Read the model definition and answer for the solid it produces. Units are mm, in the model's axes. Face numbers are marked on the shaded views. A direction names the side the tool comes from. Coordinates: 2 decimals unless noted, no trailing zeros. Loops run counter-clockwise (first coordinate to the right, second up) from the corner with the lowest first, then second, coordinate; pieces in that order, holes last. Notation, with made-up numbers: M -39,-20.5 L 12,-20.5 A21 cw 12,1.5 Z; hole C -13,-33.5 d2. An arc over 180 degrees is marked long. Use one line per item in the form item = value. Start each with the question number.
1. The part is cut by section D-D (x = -29). Give the vertices of the cut face in (y, z), plus the area to 3 significant figures.
2. Find the intervals of material crossed by probe 1 along X at (y, z) = (10.25, 8.75); probe 2 along Y at (x, z) = (-38.25, 3.5); probe 3 along X at (y, z) = (11.75, 6.5), in increasing order. Write a range as [from, to].
3. The part is cut by section B-B (x = -38.5). Give the vertices of the cut face in (y, z), plus the area to 3 significant figures.
4. The part is cut by section A-A (y = 12.5). Give the vertices of the cut face in (x, z).
5. A tool of negligible diameter and unlimited length cuts with its end or side. For the marked faces 1 and 2, from which of +Z, -Z, +X, -X, +Y, -Y can it reach the whole face along a straight path? Write none if from no direction.
6. Flat-ended cylindrical pins translate along their axes: pin 1 (2 mm diameter, centred on x = -40.5, y = 9, fed in from -Z); pin 2 (3 mm diameter, centred on y = 1.5, z = 8.5, fed in from +X); pin 3 (4.5 mm diameter, centred on x = -40.41, y = 10.65, fed in from +Z); pin 4 (2 mm diameter, centred on x = -36.5, y = 3.5, fed in from +Z). Find the tip coordinate at first contact, or state that the pin passes through.
7. For a pull along Z with two mould halves and no side action, classify the marked faces 3, 4, 5 and 6 as released by +Z, released by -Z, zero draft, split by the parting line, or undercut.
8. The part is cut by section C-C (z = 2). Give the vertices of the cut face in (x, y).
from build123d import *

# Parameters (mm, degrees)
CROQUIS1_W              = 20
CROQUIS1_H              = 17
CROQUIS1_R              = 2.5
SALIENTE_EXTRUIR2_DEPTH = 12
CORTAR_EXTRUIR2_DEPTH   = 20
CROQUIS5_R              = 3.25
CORTAR_EXTRUIR3_DEPTH   = 20
CORTAR_EXTRUIR4_START   = 4
CORTAR_EXTRUIR4_DEPTH   = 20
REDONDEO1_R             = 3


with BuildPart() as part:
    # Croquis1 → Saliente-Extruir2 (new body)
    with BuildSketch(Plane.XY):
        with Locations((-34.464447367, 6.145669291)):
            Rectangle(CROQUIS1_W, CROQUIS1_H)
        with Locations((-40.414447367, 10.645669291)):
            Circle(CROQUIS1_R, mode=Mode.SUBTRACT)
        with Locations(Location((-28.514447367, 10.645669291, 0), (0, 0, 180))):
            Circle(CROQUIS1_R, mode=Mode.SUBTRACT)
    extrude(amount=SALIENTE_EXTRUIR2_DEPTH)

    # Croquis4 → Cortar-Extruir2 (cut)
    with BuildSketch(Plane(origin=(-24.464447367, 0, 0), x_dir=(0, 0, -1), z_dir=(1, 0, 0))):
        Polygon((-12, 6.145669291), (-8.036384906, -2.354330709), (-12, -2.354330709), align=None)
    extrude(amount=-CORTAR_EXTRUIR2_DEPTH, mode=Mode.SUBTRACT)

    # Croquis5 → Cortar-Extruir3 (cut)
    with BuildSketch(Plane(origin=(0, 11.801993797, 14.637587434), x_dir=(1, 0, 0), z_dir=(0, 0.42261826174069395, -0.9063077870366525))):
        with Locations(Location((-34.464447367, 10.741063562, 0), (0, 0, 90))):
            Circle(CROQUIS5_R)
    extrude(amount=CORTAR_EXTRUIR3_DEPTH, mode=Mode.SUBTRACT)

    # Croquis6 → Cortar-Extruir4 (cut)
    with BuildSketch(Plane(origin=(0, 11.801993797, 14.637587434), x_dir=(1, 0, 0), z_dir=(0, 0.42261826174069395, -0.9063077870366525)).offset(CORTAR_EXTRUIR4_START)):
        Polygon((-29.614705106, 10.741063562), (-32.039576236, 14.941063562), (-36.889318498, 14.941063562), (-39.314189628, 10.741063562), (-36.889318498, 6.541063562), (-32.039576236, 6.541063562), align=None)
    extrude(amount=CORTAR_EXTRUIR4_DEPTH, mode=Mode.SUBTRACT)

    # Redondeo1
    # the kernel refuses this fillet: 3 mm, written as the material it takes off along each edge
    with BuildSketch(Plane(origin=(-41.464447367, 0.645669291, 3), x_dir=(0, 0, -1), z_dir=(-1, 0, 0))) as redondeo1_piece_1_section:
        Polygon((0, 0), (REDONDEO1_R, 0), (REDONDEO1_R, REDONDEO1_R), (0, REDONDEO1_R), align=None)
    redondeo1_piece_1 = extrude(amount=REDONDEO1_R, mode=Mode.PRIVATE)
    redondeo1_piece_1 = redondeo1_piece_1 - Plane(origin=(-41.464447367, 0.645669291, 3), x_dir=(0, 0.7071067811865475, 0.7071067811865475), z_dir=(-1, 0, 0)) * Sphere(REDONDEO1_R, mode=Mode.PRIVATE)
    add(redondeo1_piece_1, mode=Mode.SUBTRACT)
    with BuildSketch(Plane(origin=(-41.464447367, 0.645669291, 6.125174123), x_dir=(0, -0.422618261740694, 0.9063077870366527), z_dir=(-1, 0, 0))) as redondeo1_piece_2_section:
        Polygon((0, 0), (REDONDEO1_R, 0), (REDONDEO1_R, -REDONDEO1_R * 0.637070260807), (REDONDEO1_R * 0.422618261741, -REDONDEO1_R * 0.906307787037), align=None)
    redondeo1_piece_2 = extrude(amount=REDONDEO1_R, mode=Mode.PRIVATE)
    redondeo1_piece_2 = redondeo1_piece_2 - Plane(origin=(-41.464447367, 0.645669291, 6.125174123), x_dir=(0, 0.8433914458128839, -0.5372996083468264), z_dir=(-1, 0, 0)) * Sphere(REDONDEO1_R, mode=Mode.PRIVATE)
    add(redondeo1_piece_2, mode=Mode.SUBTRACT)
    with BuildSketch(Plane(origin=(-44.464447367, 0.645669291, 0), x_dir=(0, 0, 1), z_dir=(0, 1, 0))) as redondeo1_piece_3:
        with BuildLine():
            CenterArc((REDONDEO1_R, REDONDEO1_R), REDONDEO1_R, 180, 90)
            Line((0, REDONDEO1_R), (0, 0))
            Line((0, 0), (REDONDEO1_R, 0))
        make_face()
    extrude(amount=21.5, mode=Mode.SUBTRACT)
    with BuildSketch(Plane(origin=(-44.464447367, 14.645669291, -7.5), x_dir=(1, 0, 0), z_dir=(0, 0, 1))) as redondeo1_piece_4:
        with BuildLine():
            CenterArc((REDONDEO1_R, -REDONDEO1_R), REDONDEO1_R, 90, 90)
            Line((0, -REDONDEO1_R), (0, 0))
            Line((0, 0), (REDONDEO1_R, 0))
        make_face()
    extrude(amount=27, mode=Mode.SUBTRACT)
    with BuildSketch(Plane(origin=(-24.464447367, 14.645669291, -7.5), x_dir=(-1, 0, 0), z_dir=(0, 0, 1))) as redondeo1_piece_5:
        with BuildLine():
            CenterArc((REDONDEO1_R, REDONDEO1_R), REDONDEO1_R, 180, 90)
            Line((0, REDONDEO1_R), (0, 0))
            Line((0, 0), (REDONDEO1_R, 0))
        make_face()
    extrude(amount=27, mode=Mode.SUBTRACT)
    with BuildSketch(Plane(origin=(-24.464447367, 22.145669291, 0), x_dir=(0, 0, 1), z_dir=(0, -1, 0))) as redondeo1_piece_6:
        with BuildLine():
            CenterArc((REDONDEO1_R, REDONDEO1_R), REDONDEO1_R, 180, 90)
            Line((0, REDONDEO1_R), (0, 0))
            Line((0, 0), (REDONDEO1_R, 0))
        make_face()
    extrude(amount=32, mode=Mode.SUBTRACT)
    with BuildSketch(Plane(origin=(-16.964447367, -2.354330709, 0), x_dir=(0, 1, 0), z_dir=(-1, 0, 0))) as redondeo1_piece_7:
        with BuildLine():
            CenterArc((REDONDEO1_R, -REDONDEO1_R), REDONDEO1_R, 90, 90)
            Line((0, -REDONDEO1_R), (0, 0))
            Line((0, 0), (REDONDEO1_R, 0))
        make_face()
    extrude(amount=24.5, mode=Mode.SUBTRACT)
    with BuildSketch(Plane(origin=(-44.464447367, -2.354330709, 3), x_dir=(0, 1, 0), z_dir=(0, 0, 1))) as redondeo1_piece_8:
        with BuildLine():
            CenterArc((REDONDEO1_R, -REDONDEO1_R), REDONDEO1_R, 90, 90)
            Line((0, -REDONDEO1_R), (0, 0))
            Line((0, 0), (REDONDEO1_R, 0))
        make_face()
    extrude(amount=3.125174123, mode=Mode.SUBTRACT)
    with BuildSketch(Plane(origin=(-44.464447367, 12.942977694, 15.169636963), x_dir=(0, 0.42261826174069395, -0.9063077870366526), z_dir=(0, -0.9063077870366526, -0.42261826174069395))) as redondeo1_piece_9:
        with BuildLine():
            CenterArc((REDONDEO1_R, REDONDEO1_R), REDONDEO1_R, 180, 90)
            Line((0, REDONDEO1_R), (0, 0))
            Line((0, 0), (REDONDEO1_R, 0))
        make_face()
    extrude(amount=14.967501529, mode=Mode.SUBTRACT)
    with BuildSketch(Plane(origin=(-24.464447367, 12.942977694, 15.169636963), x_dir=(0, 0.4226182617406939, -0.9063077870366525), z_dir=(0, -0.9063077870366526, -0.42261826174069395))) as redondeo1_piece_10:
        with BuildLine():
            CenterArc((REDONDEO1_R, -REDONDEO1_R), REDONDEO1_R, 90, 90)
            Line((0, -REDONDEO1_R), (0, 0))
            Line((0, 0), (REDONDEO1_R, 0))
        make_face()
    extrude(amount=24.378712311, mode=Mode.SUBTRACT)
    with BuildSketch(Plane(origin=(-19.686420411, -2.354330709, 8.036384906), x_dir=(0, 0.9063077870366527, 0.4226182617406936), z_dir=(-1, 0, 0))) as redondeo1_piece_11:
        with BuildLine():
            CenterArc((REDONDEO1_R * 0.637070260807, REDONDEO1_R), REDONDEO1_R, 205, 65)
            Line((-REDONDEO1_R * 0.269237526229, REDONDEO1_R * 0.577381738259), (0, 0))
            Line((0, 0), (REDONDEO1_R * 0.637070260807, 0))
        make_face()
    extrude(amount=21.778026956, mode=Mode.SUBTRACT)


solid = part.part
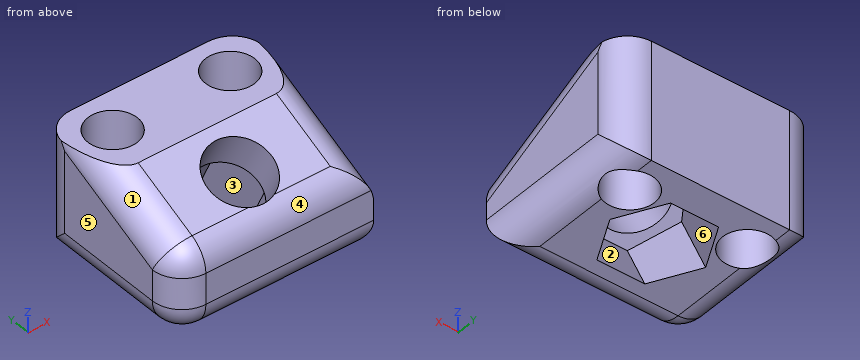
Computed values:
q1.outline = M -2.35,3 A3 ccw 0.65,0 L 8.19,0 L 8.19,12 L 6.15,12 L -0.62,8.84 A3 ccw -2.35,6.13 Z; M 13.1,0 L 14.65,0 L 14.65,12 L 13.1,12 Z
q1.area = 126 mm²
q2.probe_1 = [-44.46, -42.88], [-37.95, -30.98], [-26.05, -24.46]
q2.probe_2 = [-2.35, 3.11], [7.18, 9.39], [11.9, 14.65]
q2.probe_3 = [-44.46, -42.66], [-38.17, -30.76], [-26.27, -24.47]
q3.outline = M -2.35,3 A3 ccw 0.65,0 L 5.22,0 L 2.48,5.88 L 5.04,7.07 L 8.33,0 L 9.04,0 L 9.04,12 L 6.15,12 L -0.62,8.84 A3 ccw -2.35,6.13 Z; M 12.25,0 L 14.65,0 L 14.65,12 L 12.25,12 Z
q3.area = 126 mm²
q4.outline = M -44.34,2.15 A3 ccw -42.09,0.07 L -42.09,12 L -44.34,12 Z; M -38.74,0 L -30.19,0 L -30.19,12 L -38.74,12 Z; M -26.84,0.07 A3 ccw -24.59,2.15 L -24.59,12 L -26.84,12 Z
q5.face_1 = +Z, -X, -Y
q5.face_2 = none
q6.pin_1 = 0
q6.pin_2 = -24.48
q6.pin_3 = through
q6.pin_4 = 11.23
q7.face_3 = undercut
q7.face_4 = released by +Z
q7.face_5 = zero draft
q7.face_6 = undercut
q8.outline = M -44.29,0.65 A2.83 ccw -41.46,-2.18 L -24.64,-2.18 L -24.64,12.65 A3 ccw -27.46,14.65 L -41.46,14.65 A3 ccw -44.29,12.65 Z; hole C -40.41,10.65 d5; hole M -39.31,5.84 L -36.89,1.21 L -32.04,1.21 L -29.61,5.84 L -32.04,10.48 L -36.89,10.48 Z; hole C -28.51,10.65 d5
